For this review, use the dimensioned drawing (mm, ordinates from the lowest corner) and the shaded views. Coordinates: 2 decimals unless noted, no trailing zeros. Write each loop counter-clockwise with the first axis right and the second up, starting at its lowest first coordinate (ties: lowest second). Pieces come first, ordered by that corner, then holes. Notation, with made-up numbers: (78, -14.5) - (106, -14.5) arc R23 cw to (106, 21.5) - close; hole circle Ø2 at (82.5, 84.25). An arc over 180 degrees is marked (long way). Answer as a JSON object with one key per item and string values.
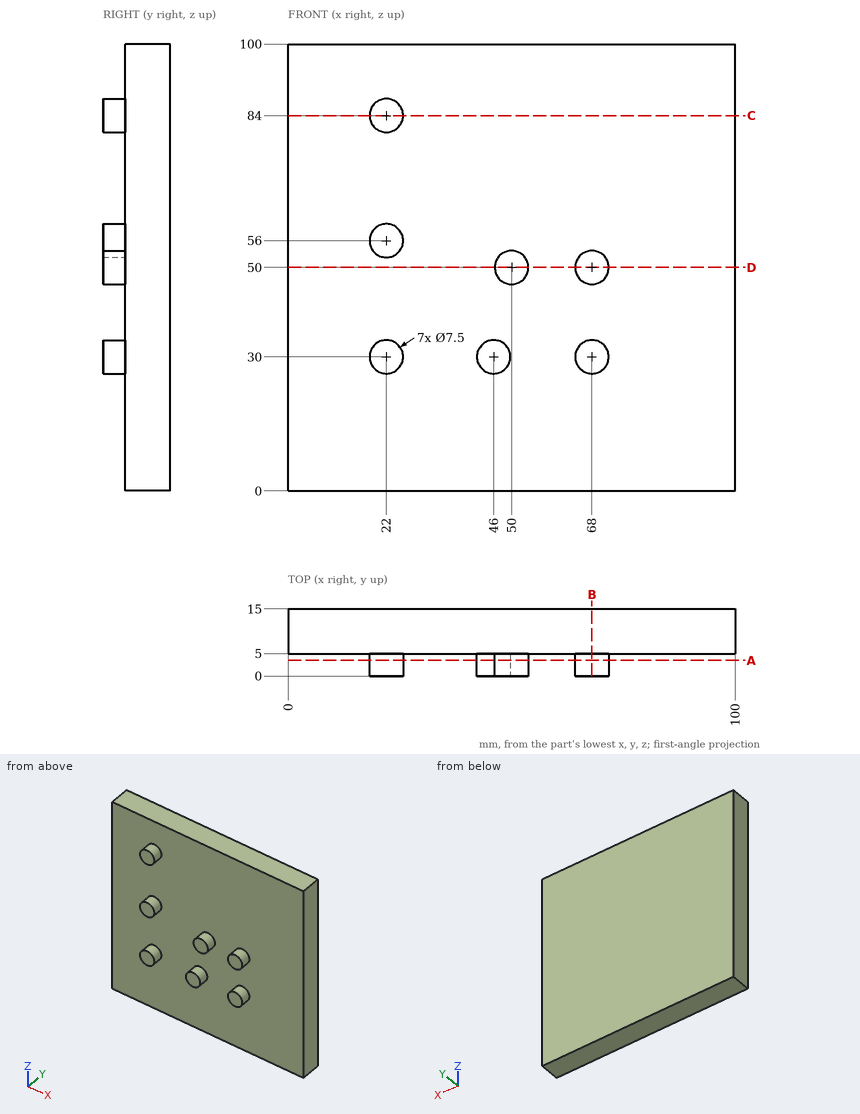
(1) Take a section at A-A, the plane y = 3.5. Write out the cut boundary in (x, z), and give its area (3 significant figures).
Solved:
{"outline": "circle Ø7.5 at (22, 30); circle Ø7.5 at (22, 56); circle Ø7.5 at (22, 84); circle Ø7.5 at (46, 30); circle Ø7.5 at (50, 50); circle Ø7.5 at (68, 30); circle Ø7.5 at (68, 50)", "area": "309 mm^2"}
(2) To check wall thickness, follow line 1 (Y direction, x = 13, z = 16); line 2 (Z direction, x = 24, y = 1.25); line 3 (Z direction, x = 68, y = 2.75). State the ranges of each line that lie inside material, in increasing order. Write a range as from..to.
Solved:
{"line 1": "y = 5..15", "line 2": "z = 26.83..33.17, 52.83..59.17, 80.83..87.17", "line 3": "z = 26.25..33.75, 46.25..53.75"}
(3) Take a section at D-D, the plane z = 50. Write out the cut boundary in (x, y).
Solved:
{"outline": "(0, 5) - (46.25, 5) - (46.25, 0) - (53.75, 0) - (53.75, 5) - (64.25, 5) - (64.25, 0) - (71.75, 0) - (71.75, 5) - (100, 5) - (100, 15) - (0, 15) - close"}
(4) Take a section at B-B, the plane x = 68. Write out the cut boundary in (y, z).
Solved:
{"outline": "(0, 26.25) - (5, 26.25) - (5, 0) - (15, 0) - (15, 100) - (5, 100) - (5, 53.75) - (0, 53.75) - (0, 46.25) - (5, 46.25) - (5, 33.75) - (0, 33.75) - close"}
(5) Take a section at C-C, the plane z = 84. Write out the cut boundary in (x, y), and give its area (3 significant figures).
Solved:
{"outline": "(0, 5) - (18.25, 5) - (18.25, 0) - (25.75, 0) - (25.75, 5) - (100, 5) - (100, 15) - (0, 15) - close", "area": "1,040 mm^2"}
(6) For pin 1 (5 mm diameter, centred on x = 53.5, y = 10, fed in from -Z); pin 2 (10 mm diameter, centred on x = 11, z = 46, fed in from -Y), all flat-tipped, find the tip position at first contact; note any pin that passes through.
Solved:
{"pin 1": "stops at z = 0", "pin 2": "stops at y = 5"}
